Source: CAD feature listing. Evaluate the final solid. Frame: model axes, mm. A direction names the side the tool comes from. Give positions to 0.01 mm unless a question says otherwise; leave off trailing zeros. Write each loop counter-clockwise with the first axis right and the second up, starting at its lowest first coordinate (ties: lowest second). Pieces come first, ordered by that corner, then holes.
Autodesk Fusion 360 part; units mm, degrees
sketch "Sketch1" plane through (0, 0, 0) normal (0, 1, 0) x (1, 0, 0)
  line L0 (0, 0) -> (28, 0)
  line L1 (28, 0) -> (28, -7)
  line L2 (28, -7) -> (13, -7)
  line L3 (13, -7) -> (13, -5)
  line L4 (13, -5) -> (26, -5)
  line L5 (26, -5) -> (26, -2)
  line L6 (26, -2) -> (2, -2)
  line L7 (2, -2) -> (2, -20)
  line L8 (2, -20) -> (0, -20)
  line L9 (0, -20) -> (0, 0)
extrude "Extrude1" add sketch "Sketch1" along normal blind 10
extrude "Extrude2" add 1 faces at (28, 3.3333, 2.3333) along direction (1, 0, 0) blind 4
extrude "Extrude3" cut 1 faces at (26, 3.3333, 4) along direction (1, 0, 0) blind 4
extrude "Extrude4" cut 1 faces at (18.6667, 3.3333, 5) along direction (0, 0, 1) blind 0.25
extrude "Extrude5" cut 1 faces at (11.3333, 3.3333, 2) along direction (0, 0, -1) blind 0.25
1. Cut plane A-A, the plane z = 5.75. Return the cut outline in (x, y).
2. Cut plane C-C, the plane y = 5. Return the cut outline in (x, z).
3. Cut plane D-D, the plane z = 9.25. Return the cut outline in (x, y), then the cut area to 3 significant figures.
4. Cut plane B-B, the plane x = 27.5. Return the cut outline in (y, z).
5. Contact query for flat-ended pins moving along their axis: P1, Ø1.4, axis at y = 5.5, z = 6, coming from the -X side; P2, Ø3, axis at x = 10, y = 7, coming from the +Z side; P3, Ø3, axis at y = 4.5, z = 10.5, coming from the +X side. Output: stop coordinate, or through.
6. Access query for faces 1 (the flat face through (1, 5, 20)), 2 (the flat face through (30, 5, 3)), 3 (the flat face through (2, 5, 11)), 4 (the flat face through (14, 10, 6)), 5 (the flat face through (23, 5, 7)). Directions: +Z, -Z, +X, -X, +Y, -Y. A direction counts if a zero-diameter tool reaches every point of the face in a straight line with its end or side. Return the directions, or none.
7. Mould query, pull axis X, two halves, no side actions, for faces 6 (the flat face through (16, 5, 0)), 7 (the flat face through (32, 5, 3)), 8 (the flat face through (13, 5, 6)). Classes: +X half, -X half, draft (parallel to the pull), parting line (faces both ways), or undercut.
8. Line query: L1, parallel to X at y = 4.25, z = 2.25; L2, parallel to Z at x = 17.5, y = 3; L3, parallel to X at y = 3.5, z = 5.5. Output: solid intervals per line, ascending.
Response values:
1. outline: (0, 0) - (2, 0) - (2, 10) - (0, 10) - close; (13, 0) - (32, 0) - (32, 10) - (13, 10) - close
2. outline: (0, 0) - (32, 0) - (32, 7) - (13, 7) - (13, 5.25) - (30, 5.25) - (30, 1.75) - (2, 1.75) - (2, 20) - (0, 20) - close
3. outline: (0, 0) - (2, 0) - (2, 10) - (0, 10) - close
3. area: 20.0 mm2
4. outline: (0, 0) - (10, 0) - (10, 1.75) - (0, 1.75) - close; (0, 5.25) - (10, 5.25) - (10, 7) - (0, 7) - close
5. P1: stops at x = 0
5. P2: stops at z = 1.75
5. P3: stops at x = 2
6. face 1: +Z, +X, -X, +Y, -Y
6. face 2: +Y, -Y
6. face 3: +Z, +Y, -Y
6. face 4: +Z, -Z, +X, -X, +Y
6. face 5: +Z, +X, +Y, -Y
7. face 6: draft
7. face 7: +X half
7. face 8: undercut
8. L1: x = 0 to 2, 30 to 32
8. L2: z = 0 to 1.75, 5.25 to 7
8. L3: x = 0 to 2, 13 to 32
